from build123d import *

# Parameters (mm, degrees)
PAD_DEPTH    = 10
PAD001_DEPTH = 25
PAD002_DEPTH = 25
FILLET_R     = 3
FILLET001_R  = 3
FILLET002_R  = 3
FILLET003_R  = 3
FILLET004_R  = 3
FILLET005_R  = 3
FILLET006_R  = 3
FILLET007_R  = 3


with BuildPart() as part:
    # Sketch → Pad (new body)
    with BuildSketch(Plane.XY):
        Polygon((0, 0), (25, 0), (25, 62.5), (225, 62.5), (225, 0), (250, 0), (250, 150), (225, 150), (225, 87.5), (25, 87.5), (25, 150), (0, 150), align=None)
    extrude(amount=PAD_DEPTH)

    # Sketch001 → Pad001 (join)
    with BuildSketch(Plane.YZ):
        Polygon((17.5, 0), (62.5, 60), (62.5, 0), align=None)
        Polygon((86.5, 0), (86.5, 60), (131.5, 0), align=None)
    extrude(amount=PAD001_DEPTH)

    # Sketch002 (on Face23 of Pad001) → Pad002 (join)
    with BuildSketch(Plane.YZ.offset(250)):
        Polygon((17.5, 0), (62.5, 60), (62.5, 0), align=None)
        Polygon((86.5, 60), (86.5, 0), (131.5, 0), align=None)
    extrude(amount=-PAD002_DEPTH)

    # Fillet
    fillet_edges = [part.edges().sort_by_distance(p)[0] for p in [
        (237.5, 150, 10),
    ]]
    fillet(fillet_edges, radius=FILLET_R)

    # Fillet001
    fillet001_edges = [part.edges().sort_by_distance(p)[0] for p in [
        (12.5, 150, 10),
    ]]
    fillet(fillet001_edges, radius=FILLET001_R)

    # Fillet002
    fillet002_edges = [part.edges().sort_by_distance(p)[0] for p in [
        (237.5, 0, 10),
    ]]
    fillet(fillet002_edges, radius=FILLET002_R)

    # Fillet003
    fillet003_edges = [part.edges().sort_by_distance(p)[0] for p in [
        (12.5, 0, 10),
    ]]
    fillet(fillet003_edges, radius=FILLET003_R)

    # Fillet004
    fillet004_edges = [part.edges().sort_by_distance(p)[0] for p in [
        (237.5, 86.5, 60),
    ]]
    fillet(fillet004_edges, radius=FILLET004_R)

    # Fillet005
    fillet005_edges = [part.edges().sort_by_distance(p)[0] for p in [
        (237.5, 62.5, 60),
    ]]
    fillet(fillet005_edges, radius=FILLET005_R)

    # Fillet006
    fillet006_edges = [part.edges().sort_by_distance(p)[0] for p in [
        (12.5, 86.5, 60),
    ]]
    fillet(fillet006_edges, radius=FILLET006_R)

    # Fillet007
    fillet007_edges = [part.edges().sort_by_distance(p)[0] for p in [
        (12.5, 62.5, 60),
    ]]
    fillet(fillet007_edges, radius=FILLET007_R)


solid = part.part
The model under review builds one solid part; all positions refer to its coordinate system, in mm. A direction names the side the tool comes from. Round coordinates to 2 decimals unless told otherwise and drop trailing zeros. Loops run counter-clockwise (first coordinate to the right, second up) from the corner with the lowest first, then second, coordinate; pieces in that order, holes last. Notation, with made-up numbers: (-29, -33) -> (29, -33) arc R20 ccw to (29, -8) -> close; hole circle Ø4 at (32, 22.5). An arc over 180 degrees is marked (long way). Answer as CSV lines item,"result".
1) Add section A-A on y = 110.5. Write out the cut boundary in (x, z), plus the area to 3 significant figures.
Geometry results:
outline,"(0, 0) -> (25, 0) -> (25, 28) -> (0, 28) -> close; (225, 0) -> (250, 0) -> (250, 28) -> (225, 28) -> close"
area,"1,400 mm²"
2) Add section D-D on z = 14.5. Write out the cut boundary in (x, y) (3 decimals), plus the area to 3 significant figures.
Geometry results:
outline,"(0, 28.375) -> (25, 28.375) -> (25, 62.5) -> (0, 62.5) -> close; (0, 86.5) -> (25, 86.5) -> (25, 120.625) -> (0, 120.625) -> close; (225, 28.375) -> (250, 28.375) -> (250, 62.5) -> (225, 62.5) -> close; (225, 86.5) -> (250, 86.5) -> (250, 120.625) -> (225, 120.625) -> close"
area,"3,410 mm²"
3) For P1, Ø11, axis at x = 241, y = 19, coming from the +Z side; P2, Ø7.5, axis at x = 242, z = 25, coming from the +Y side; P3, Ø7.5, axis at x = 8.5, z = 36, coming from the -Y side; P4, Ø1, axis at x = 50.5, z = 12, coming from the +Y side, all flat-tipped, find the tip position at first contact; note any pin that passes through.
Geometry results:
P1,"stops at z = 10"
P2,"stops at y = 115.56"
P3,"stops at y = 41.69"
P4,"passes through"
4) Draft analysis for pull direction Y (two halves, no side actions). For faces 1 (the face through (123, 75, 10)), 2 (the face through (237, 136, 10)), 3 (the face through (124, 62.5, 5)), state which applies: pulls with the +Y half, pulls with the -Y half, needs draft (parallel to the pull), parting line crosses it, or undercut.
Geometry results:
face 1,"undercut"
face 2,"needs draft"
face 3,"pulls with the -Y half"
5) To check wall thickness, follow line 1 along Z through (x, y) = (22, 128); line 2 along X through (y, z) = (53, 32); line 3 along Y through (x, z) = (11.5, 30). State the ranges of each line that lie inside material, in increasing order. Write a range as from..to.
Geometry results:
line 1,"z = 0..10"
line 2,"x = 0..25, 225..250"
line 3,"y = 40..62.5, 86.5..109"
6) Add section B-B on z = 41. Write out the cut boundary in (x, y).
Geometry results:
outline,"(0, 48.25) -> (25, 48.25) -> (25, 62.5) -> (0, 62.5) -> close; (0, 86.5) -> (25, 86.5) -> (25, 100.75) -> (0, 100.75) -> close; (225, 48.25) -> (250, 48.25) -> (250, 62.5) -> (225, 62.5) -> close; (225, 86.5) -> (250, 86.5) -> (250, 100.75) -> (225, 100.75) -> close"
7) Add section C-C on y = 128. Write out the cut boundary in (x, z).
Geometry results:
outline,"(0, 0) -> (25, 0) -> (25, 10) -> (0, 10) -> close; (225, 0) -> (250, 0) -> (250, 10) -> (225, 10) -> close"
8) Tool access review of faces 4 (the face through (12, 86.5, 30)), 5 (the face through (12, 14, 10)), 6 (the face through (12, 136, 10)): name each direction out of +Z, -Z, +X, -X, +Y, -Y from which nothing blocks a thin tool from reaching the whole face with its end or side.
Geometry results:
face 4,"+Z, +X, -X"
face 5,"+Z, +X, -X, -Y"
face 6,"+Z, +X, -X, +Y"
